Geometry check sheet. Reference: the model listing, model coordinates, mm. A direction names the side the tool comes from. Round coordinates to 2 decimals unless told otherwise and drop trailing zeros. Write each loop counter-clockwise with the first axis right and the second up, starting at its lowest first coordinate (ties: lowest second). Pieces come first, ordered by that corner, then holes. Notation, with made-up numbers: (79, 37) -> (120, 37) arc R14 cw to (120, 62) -> close; hole circle Ø7 at (-5, 58). An arc over 180 degrees is marked (long way). Return JSON: item names as keys, results as strings. Group by question number.
from build123d import *

# Parameters (mm, degrees)
F0_R      = 6.35
F1_DEPTH  = 25.4
F2_R      = 9.525
F3_DEPTH  = 9.8425
F4_R      = 1.5875
F6_DEPTH  = 6.35
F8_R      = 9.525
F9_DEPTH  = 9.779
F10_R     = 1.5875
F12_DEPTH = 6.35


with BuildPart() as f1:
    # F0 (on Top) → F1 (new body)
    with BuildSketch(Plane.XY):
        Circle(F0_R)
    extrude(amount=F1_DEPTH)

    # F8 (on face) → F9 (join)
    with BuildSketch(Plane.XY.offset(25.4)):
        Circle(F8_R)
    extrude(amount=F9_DEPTH)

    # F10
    f10_edges = [f1.edges().sort_by_distance(p)[0] for p in [
        (-9.525, 0, 35.179),
    ]]
    fillet(f10_edges, radius=F10_R)

    # F11 (on face) → F12 (cut)
    with BuildSketch(Plane.XY.offset(35.179)):
        Polygon((1.58678, -6.254315), (6.209785, -1.752966), (4.623006, 4.501349), (-1.58678, 6.254315), (-6.209785, 1.752966), (-4.623006, -4.501349), align=None)
    extrude(amount=-F12_DEPTH, mode=Mode.SUBTRACT)


with BuildPart() as f3:
    # F2 (on face) → F3 (new body)
    with BuildSketch(Plane.XY.offset(25.4)):
        Circle(F2_R)
    extrude(amount=F3_DEPTH)

    # F4
    f4_edges = [f3.edges().sort_by_distance(p)[0] for p in [
        (-9.525, 0, 35.2425),
    ]]
    fillet(f4_edges, radius=F4_R)

    # F5 (on face) → F6 (cut)
    with BuildSketch(Plane.XY.offset(35.2425)):
        Polygon((6.020851, -2.017882), (4.757963, 4.205269), (-1.262889, 6.223151), (-6.020851, 2.017882), (-4.757963, -4.205269), (1.262889, -6.223151), align=None)
    extrude(amount=-F6_DEPTH, mode=Mode.SUBTRACT)


solid = f1.part
1) Mould release check, pull along X, two halves, no side actions. Record for faces 4 (the face through (3.9, -4, 32)), 5 (the face through (0, 0, 0)), 6 (the face through (-1.38, -6.2, 12.52)): +X half, -X half, draft (parallel to the pull), parting line (faces both ways), or undercut.
2) Tool access check on faces 1 (the face through (0, 0, 28.829)), 2 (the face through (2, -6.2, 25.4)), 3 (the face through (3.4, -5.2, 35.179)). Record the directions out of +Z, -Z, +X, -X, +Y, -Y that give a thin tool (end or side, any length) a straight path to the whole face; none if there is none.
3) Sectioned sample at A-A on z = 31. Enter the section's corners in (x, y) (3 decimals).
4) Sectioned sample at C-C on z = 8.5. Enter the section's corners in (x, y), and give its area (3 significant figures).
5) Go/stop test with flat-tipped pins: P1, Ø1, axis at x = -7, z = 31, coming from the -Y side; P2, Ø6, axis at x = -5.5, y = -2.5, coming from the -Z side; P3, Ø5, axis at y = -2.5, z = 8.5, coming from the +X side; P4, Ø4, axis at x = -3.5, z = 25.5, coming from the -Y side. Record where each tip stops, or that it passes through.
6) Material ranges on probe 1 along Z at (x, y) = (1, -4); probe 2 along X at (y, z) = (0.25, 19), recorded low to high. Write a range as [from, to].
Evaluation:
{
 "1": {"face 4": "undercut", "face 5": "draft", "face 6": "parting line"},
 "2": {"face 1": "+Z", "face 2": "-Z", "face 3": "+Z, +X, -X, +Y, -Y"},
 "3": {"outline": "circle Ø19.05 at (0, 0); hole (-6.21, 1.753) -> (-4.623, -4.501) -> (1.587, -6.254) -> (6.21, -1.753) -> (4.623, 4.501) -> (-1.587, 6.254) -> close"},
 "4": {"outline": "circle Ø12.7 at (0, 0)", "area": "127 mm2"},
 "5": {"P1": "stops at y = -6.96", "P2": "stops at z = 0", "P3": "stops at x = 6.35", "P4": "stops at y = -9.41"},
 "6": {"probe 1": "z = [0, 28.83]", "probe 2": "x = [-6.35, 6.35]"}
}
